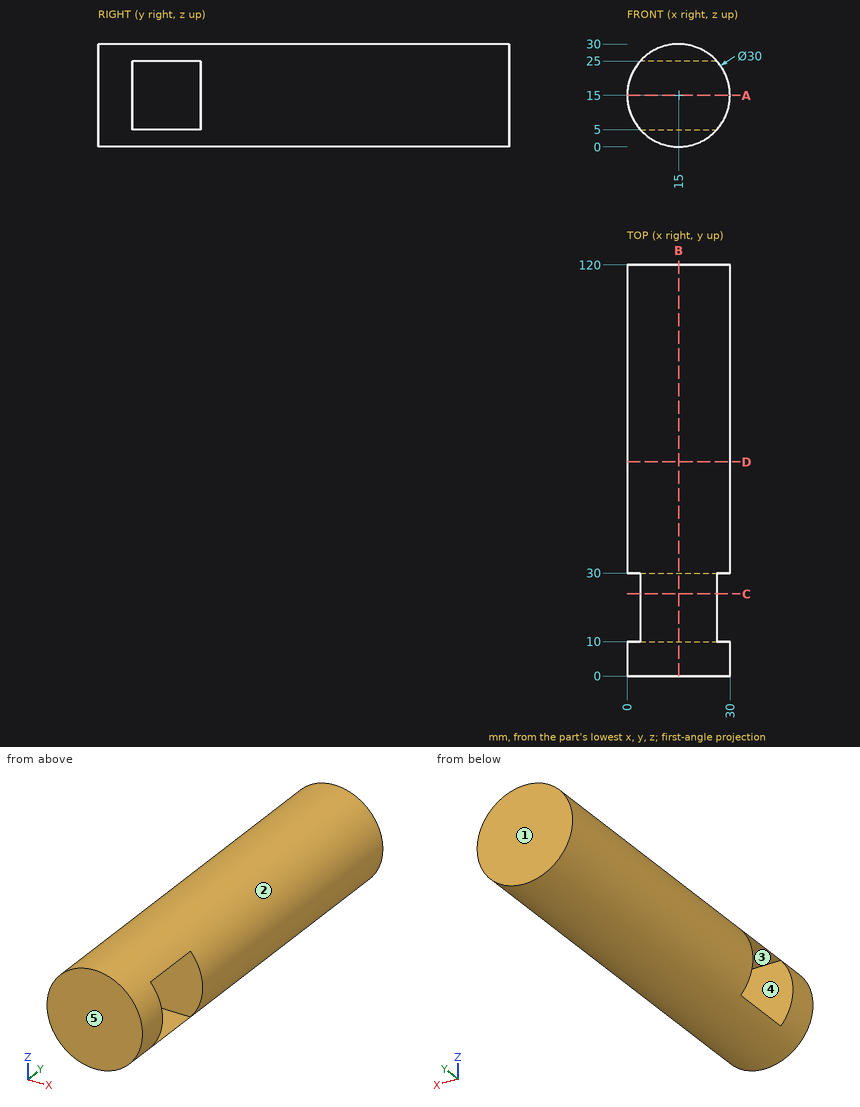
Could you check a few things on this drawing? It's one solid part, dimensions in mm from its lowest x, y, z. A direction names the side the tool comes from. Round coordinates to 2 decimals unless told otherwise and drop trailing zeros. Order: outer loops, then holes, each group sorted by start corner. A loop starts at its lowest first (then second) coordinate and runs counter-clockwise, first axis right, second up.
(1) I'm going to push flat-ended pins straight in: pin 1 (8 mm diameter, centred on y = 79.5, z = 8, fed in from -X); pin 2 (10 mm diameter, centred on y = 76.5, z = 4.5, fed in from -X); pin 3 (3 mm diameter, centred on x = 5, y = 79.5, fed in from -Z); pin 4 (1.5 mm diameter, centred on y = 18, z = 24, fed in from +X). Where does each tip first touch, or does it pass through?
Response values:
pin 1: stops at x = 0.3
pin 2: stops at x = 1.04
pin 3: stops at z = 2.64
pin 4: passes through
(2) Imagine slicing it at C-C (y = 24). Write out the boundary of the cut face in (x, z), plus the area to 3 significant figures.
Response values:
outline: (3.82, 5) arc R15 ccw to (26.18, 5) - close; (3.82, 25) - (26.18, 25) arc R15 ccw to start
area: 155 mm2
(3) Imagine slicing it at D-D (y = 62.5). Write out the boundary of the cut face in (x, z).
Response values:
outline: circle Ø30 at (15, 15)
(4) Which directions (+Z, -Z, +X, -X, +Y, -Y) give clear straight access to the entire face, cutting with the end or side of a thin tool? Please do the marked faces 4 and 5.
Response values:
face 4: +X, -X
face 5: +Z, -Z, +X, -X, -Y
(5) Please list where these lines run through material, in increasing order: line 1 along Y through (x, z) = (12.5, 21.25); line 2 along Z through (x, y) = (25, 47); line 3 along Z through (x, y) = (15.25, 48.5).
Response values:
line 1: y = 0 to 10, 30 to 120
line 2: z = 3.82 to 26.18
line 3: z = 0 to 30
(6) Imagine slicing it at B-B (x = 15). Write out the boundary of the cut face in (y, z), plus the area to 3 significant figures.
Response values:
outline: (0, 0) - (120, 0) - (120, 30) - (0, 30) - close; hole (10, 5) - (30, 5) - (30, 25) - (10, 25) - close
area: 3,200 mm2
(7) If we mould it in two halves opening along Z, with no side actions, what happens to the marked faces 1, 2 and 3? For each: released by +Z, released by -Z, zero draft, split by the parting line, or undercut.
Response values:
face 1: zero draft
face 2: split by the parting line
face 3: undercut
(8) Imagine slicing it at A-A (z = 15). Write out the boundary of the cut face in (x, y), plus the area to 3 significant figures.
Response values:
outline: (0, 0) - (30, 0) - (30, 10) - (0, 10) - close; (0, 30) - (30, 30) - (30, 120) - (0, 120) - close
area: 3,000 mm2
